Check sheet for the modelled part. Datum: model origin and axes. Units: mm. Face numbers are marked on the shaded views. A direction names the side the tool comes from. Round coordinates to 2 decimals unless told otherwise and drop trailing zeros. Loops run counter-clockwise (first coordinate to the right, second up) from the corner with the lowest first, then second, coordinate; pieces in that order, holes last. Notation, with made-up numbers: (16, 27.5) - (73, 27.5) arc R12 ccw to (73, 35.5) - close; hole circle Ø3 at (-21, -28). An arc over 180 degrees is marked (long way). Return JSON: item names as keys, results as strings.
Autodesk Inventor part; units mm, degrees
ref_plane "YZ Plane" through (0, 0, 0) normal (1, 0, 0) x (0, 1, 0)
ref_plane "XZ Plane" through (0, 0, 0) normal (0, 1, 0) x (-1, 0, 0)
ref_plane "XY Plane" through (0, 0, 0) normal (0, 0, 1) x (1, 0, 0)
sketch "Sketch1" plane through (0, 0, 0) normal (0, 0, 1) x (1, 0, 0)
  line L0 (22.9, 0.025) -> (-22.9, 0.025)
  line L1 (22.9, 42.1) -> (22.9, 0.025)
  line L2 (22.9, 42.1) -> (17.05, 42.1)
  line L3 (17.05, 7.7) -> (17.05, 42.1)
  line L4 (-17.05, 7.7) -> (17.05, 7.7)
  line L5 (-17.05, 7.7) -> (-17.05, 42.1)
  line L6 (-17.05, 42.1) -> (-22.9, 42.1)
  line L7 (-22.9, 0.025) -> (-22.9, 42.1)
  circle A0 centre (19.9, 34.8) radius 2.0625
  circle A1 centre (-19.9, 34.8) radius 2.0625
  circle A2 centre (19.9, 15) radius 2.0625
  circle A3 centre (-19.9, 15) radius 2.0625
  circle A4 centre (10, 3.85) radius 1.5625
  circle A5 centre (-10, 3.85) radius 1.5625
  line L8 (-17.05, 7.7) -> (17.05, 7.7)
  line L9 (17.05, 7.7) -> (17.05, 42.1)
  line L10 (17.05, 42.1) -> (-17.05, 42.1)
  line L11 (-17.05, 42.1) -> (-17.05, 7.7)
  line L12 (-17.55, 47.6) -> (17.55, 47.6)
  line L13 (22.55, 42.6) -> (22.55, 7.2)
  line L14 (17.55, 2.2) -> (-17.55, 2.2)
  line L15 (-22.55, 7.2) -> (-22.55, 42.6)
  line L16 (-22.55, 24.9) -> (22.55, 24.9)
  circle A6 centre (0, 24.9) radius 12.75
  arc A7 (-17.55, 47.6) -> (-22.55, 42.6) centre (-17.55, 42.6) ccw
  arc A8 (22.55, 42.6) -> (17.55, 47.6) centre (17.55, 42.6) ccw
  arc A9 (17.55, 2.2) -> (22.55, 7.2) centre (17.55, 7.2) ccw
  arc A10 (-22.55, 7.2) -> (-17.55, 2.2) centre (-17.55, 7.2) ccw
  point P0 (0, 0)
  dimension "d0" = 5.5
  dimension "d1" = 25.5
  dimension "d2" = 5
extrude "Extrusion1" add sketch "Sketch1" along normal mid plane 5 contours L13 L16 L3 L2 | L2 L10 L6 L15 A7 L12 A8 L13 | L6 L5 L16 L15 | L3 L16 A6 L5 L10 | L13 A9 L14 A10 L15 L16 L5 L4 L3 | L3 L4 L5 L16 A6 | A0 | A1 | A2 | A3 | A4 | A5
sketch "Sketch2" plane through (0, 0, 2.5) normal (0, 0, 1) x (1, 0, 0)
  line L0 (22.9, 0.025) -> (-22.9, 0.025)
  line L1 (22.9, 42.1) -> (22.9, 0.025)
  line L2 (22.9, 42.1) -> (17.05, 42.1)
  line L3 (17.05, 7.7) -> (17.05, 42.1)
  line L4 (-17.05, 7.7) -> (17.05, 7.7)
  line L5 (-17.05, 7.7) -> (-17.05, 42.1)
  line L6 (-17.05, 42.1) -> (-22.9, 42.1)
  line L7 (-22.9, 0.025) -> (-22.9, 42.1)
  circle A0 centre (19.9, 34.8) radius 2.0625
  circle A1 centre (-19.9, 34.8) radius 2.0625
  circle A2 centre (19.9, 15) radius 2.0625
  circle A3 centre (-19.9, 15) radius 2.0625
  circle A4 centre (10, 3.85) radius 1.5625
  circle A5 centre (-10, 3.85) radius 1.5625
  point P0 (0, 0)
extrude "Extrusion2" add sketch "Sketch2" along normal blind 2.5 contours A0 | A1 | A2 | A3
chamfer "Chamfer1" distance 2.5 angle 3.75 1 edges at (17.8375, 34.8, 5) measured on face at (21.7975, 35.6084, 4.1667)
chamfer "Chamfer2" distance 2.5 angle 3.75 1 edges at (17.8375, 15, 5) measured on face at (21.9358, 14.6692, 4.1667)
chamfer "Chamfer3" distance 2.5 angle 3.75 1 edges at (-21.9625, 34.8, 5) measured on face at (-18.0025, 35.6084, 4.1667)
chamfer "Chamfer4" distance 2.5 angle 3.75 1 edges at (-21.9625, 15, 5) measured on face at (-17.8642, 14.6692, 4.1667)
properties part number "Filter Mount"
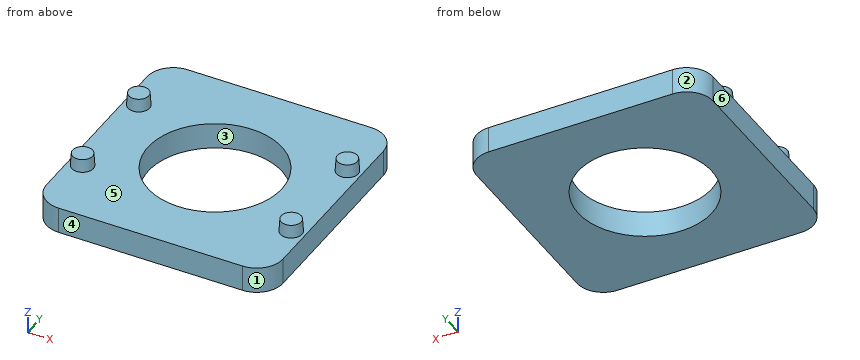
Q1. Draft check along X on the marked faces 1, 2, 3 and 4. Enter one of: released by +X, released by -X, zero draft, split by the parting line, or undercut.
Answer key:
{"face 1": "released by +X", "face 2": "released by -X", "face 3": "undercut", "face 4": "zero draft"}
Q2. Sectioned sample at D-D (z = 3.5). Enter the section's corners in (x, y).
Answer key:
{"outline": "circle Ø3.99 at (-19.9, 15); circle Ø3.99 at (-19.9, 34.8); circle Ø3.99 at (19.9, 15); circle Ø3.99 at (19.9, 34.8)"}
Q3. Scan lines: probe 1 along X at (y, z) = (24.9, 1.4); probe 2 along Y at (x, z) = (0, -0.75); probe 3 along Y at (x, z) = (-8, -1.5). Record each from-to range of solid material in increasing order. Write a range as [from, to].
Answer key:
{"probe 1": "x = [-22.55, -12.75], [12.75, 22.55]", "probe 2": "y = [2.2, 12.15], [37.65, 47.6]", "probe 3": "y = [2.2, 14.97], [34.83, 47.6]"}
Q4. Sectioned sample at B-B (z = -1). Enter the section's corners in (x, y).
Answer key:
{"outline": "(-22.55, 7.2) arc R5 ccw to (-17.55, 2.2) - (17.55, 2.2) arc R5 ccw to (22.55, 7.2) - (22.55, 42.6) arc R5 ccw to (17.55, 47.6) - (-17.55, 47.6) arc R5 ccw to (-22.55, 42.6) - close; hole circle Ø25.5 at (0, 24.9)"}
Q5. Tool access check on the marked faces 5 and 6. Record the directions out of +Z, -Z, +X, -X, +Y, -Y that give a thin tool (end or side, any length) a straight path to the whole face; none if there is none.
Answer key:
{"face 5": "+Z", "face 6": "+Z, -Z, -X, +Y, -Y"}
Q6. Sectioned sample at A-A (x = 0). Enter the section's corners in (y, z), plus the area to 3 significant figures.
Answer key:
{"outline": "(2.2, -2.5) - (12.15, -2.5) - (12.15, 2.5) - (2.2, 2.5) - close; (37.65, -2.5) - (47.6, -2.5) - (47.6, 2.5) - (37.65, 2.5) - close", "area": "99.5 mm²"}
Q7. Depth check by flat-ended pin: P1, Ø2, axis at x = -0.5, y = 8, coming from the +Z side. Enter the tip coordinate at first touch or a pass-through.
Answer key:
{"P1": "stops at z = 2.5"}
